The listing builds one solid part. Answer for the finished solid, in the listing's coordinates (mm). A direction names the side the tool comes from. Coordinates: 2 decimals unless noted, no trailing zeros. Write each loop counter-clockwise with the first axis right and the second up, starting at its lowest first coordinate (ties: lowest second). Pieces come first, ordered by that corner, then holes.
from build123d import *

# Parameters (mm, degrees)
BOSS_EXTRUDE1_DEPTH        = 58
SKETCH3_OUTSIDE_W          = 147.986
SKETCH3_OUTSIDE_H          = 126.948
TAB_AND_SLOT_CONTOUR_DEPTH = 3
MOUNTING_TAB_SLOTS_REACH   = 197.382
SKETCH4_W                  = 10.2
SKETCH4_H                  = 4.48444402


with BuildPart() as part:
    # Sketch1 → Boss-Extrude1 (new, symmetric)
    with BuildSketch(Plane.XY):
        Polygon((-63.840100917, 220.738237129), (-95.659428373, 133.315353441), (-98.478506236, 134.341413871), (-66.659178779, 221.764297559), align=None)
    extrude(amount=BOSS_EXTRUDE1_DEPTH, both=True)

    # Sketch3 outside → tab and slot contour (cut)
    with BuildSketch(Plane(origin=(-130.135207504, 47.365341962, 0), x_dir=(0, 0, 1), z_dir=(-0.9396926207859098, 0.3420201433256651, 0))):
        with Locations((0, 139.075)):
            Rectangle(SKETCH3_OUTSIDE_W, SKETCH3_OUTSIDE_H)
        with BuildLine():
            Line((-44.02892944, 185.59149209), (44.02892944, 185.59149209))
            ThreePointArc((44.02892944, 185.59149209), (47.369183029, 184.312070804), (49, 181.128574477))
            Line((49, 181.128574477), (57.97107056, 98.09508485))
            ThreePointArc((57.97107056, 98.09508485), (56.720578714, 94.217748875), (53, 92.558002463))
            Line((53, 92.558002463), (-53, 92.558002463))
            ThreePointArc((-53, 92.558002463), (-56.720578714, 94.217748875), (-57.97107056, 98.09508485))
            Line((-57.97107056, 98.09508485), (-49, 181.128574477))
            ThreePointArc((-49, 181.128574477), (-47.369183029, 184.312070804), (-44.02892944, 185.59149209))
        make_face(mode=Mode.SUBTRACT)
    extrude(amount=-TAB_AND_SLOT_CONTOUR_DEPTH, mode=Mode.SUBTRACT)

    # Sketch4 → mounting tab slots (cut, up to next)
    with BuildSketch(Plane(origin=(-130.135207504, 47.365341962, 0), x_dir=(0, 0, 1), z_dir=(-0.9396926207859099, 0.3420201433256647, 0)), mode=Mode.PRIVATE) as mounting_tab_slots_sk1:
        with Locations((-25, 173.44927008)):
            Rectangle(SKETCH4_W, SKETCH4_H)
    mounting_tab_slots_tool1 = extrude(mounting_tab_slots_sk1.sketch, amount=-MOUNTING_TAB_SLOTS_REACH, mode=Mode.PRIVATE) & part.part
    # Sketch4 → mounting tab slots (cut, up to next)
    with BuildSketch(Plane(origin=(-130.135207504, 47.365341962, 0), x_dir=(0, 0, 1), z_dir=(-0.9396926207859099, 0.3420201433256647, 0)), mode=Mode.PRIVATE) as mounting_tab_slots_sk2:
        with Locations((-25, 103.608313771)):
            Rectangle(SKETCH4_W, SKETCH4_H)
    mounting_tab_slots_tool2 = extrude(mounting_tab_slots_sk2.sketch, amount=-MOUNTING_TAB_SLOTS_REACH, mode=Mode.PRIVATE) & part.part
    # Sketch4 → mounting tab slots (cut, up to next)
    with BuildSketch(Plane(origin=(-130.135207504, 47.365341962, 0), x_dir=(0, 0, 1), z_dir=(-0.9396926207859099, 0.3420201433256647, 0)), mode=Mode.PRIVATE) as mounting_tab_slots_sk3:
        with Locations((25, 173.44927008)):
            Rectangle(SKETCH4_W, SKETCH4_H)
    mounting_tab_slots_tool3 = extrude(mounting_tab_slots_sk3.sketch, amount=-MOUNTING_TAB_SLOTS_REACH, mode=Mode.PRIVATE) & part.part
    # Sketch4 → mounting tab slots (cut, up to next)
    with BuildSketch(Plane(origin=(-130.135207504, 47.365341962, 0), x_dir=(0, 0, 1), z_dir=(-0.9396926207859099, 0.3420201433256647, 0)), mode=Mode.PRIVATE) as mounting_tab_slots_sk4:
        with Locations((25, 103.608313771)):
            Rectangle(SKETCH4_W, SKETCH4_H)
    mounting_tab_slots_tool4 = extrude(mounting_tab_slots_sk4.sketch, amount=-MOUNTING_TAB_SLOTS_REACH, mode=Mode.PRIVATE) & part.part
    add(mounting_tab_slots_tool1.solids().sort_by_distance((-70.812063, 210.354341, -25))[0], mode=Mode.SUBTRACT)
    add(mounting_tab_slots_tool2.solids().sort_by_distance((-94.699077, 144.72531, -25))[0], mode=Mode.SUBTRACT)
    add(mounting_tab_slots_tool3.solids().sort_by_distance((-70.812063, 210.354341, 25))[0], mode=Mode.SUBTRACT)
    add(mounting_tab_slots_tool4.solids().sort_by_distance((-94.699077, 144.72531, 25))[0], mode=Mode.SUBTRACT)


solid = part.part
Q1. The part is cut by section C-C, the plane x = -83. Write down the section's boundary in (y, z).
Answers below:
outline: (168.1, -54.57) - (176.87, -53.68) - (176.87, 53.68) - (168.1, 54.57) - close
Q2. Given pin 1 (5 mm diameter, centred on x = -94, y = 144.5, fed in from -Z); pin 2 (2 mm diameter, centred on x = -94, y = 144.5, fed in from +Z); pin 3 (5 mm diameter, centred on y = 207, z = -44.5, fed in from -X), each flat-ended and moving along its own axis, determine where each tip first touches the part or whether it passes through.
Answers below:
pin 1: stops at z = -57.64
pin 2: stops at z = 57.48
pin 3: stops at x = -72.94
Q3. Find the intervals of material crossed by probe 1 along Z at (x, y) = (-93, 142); probe 2 along X at (y, z) = (192, 44); probe 3 along X at (y, z) = (144, -32.5), in increasing order.
Answers below:
probe 1: z = -57.59 to -30.1, -19.9 to 19.9, 30.1 to 57.59
probe 2: x = -77.49 to -74.3
probe 3: x = -94.96 to -91.77
Q4. Which of the six approach directions +Z, -Z, +X, -X, +Y, -Y give full straight-line access (tool end or side, diameter ignored) to faces 1 (the face through (-80.797, 178.598, 53.423)), 2 (the face through (-81.194, 177.506, -53.548)), 3 (the face through (-68.655, 211.955, 24.929)), 4 (the face through (-94.076, 142.112, 24.929)), 5 (the face through (-93, 144, -30.1))?
Answers below:
face 1: +Z, +X, +Y
face 2: -Z, +X, +Y
face 3: -X
face 4: +X
face 5: none
Q5. The part is cut by section D-D, the plane z = -6.5. Write down the section's boundary in (x, y), then the cut area to 3 significant figures.
Answers below:
outline: (-98.48, 134.34) - (-95.66, 133.32) - (-63.84, 220.74) - (-66.66, 221.76) - close
area: 279 mm2
Q6. The part is cut by section B-B, the plane y = 210. Write down the section's boundary in (x, z).
Answers below:
outline: (-70.94, -49.87) - (-67.75, -49.75) - (-67.75, -30.1) - (-70.94, -30.1) - close; (-70.94, -19.9) - (-67.75, -19.9) - (-67.75, 19.9) - (-70.94, 19.9) - close; (-70.94, 30.1) - (-67.75, 30.1) - (-67.75, 49.75) - (-70.94, 49.87) - close
Q7. Determine the mould class of faces 6 (the face through (-92.542, 146.326, -25.071)), 7 (the face through (-97.089, 133.836, 0.742)), 8 (the face through (-82.79, 177.44, 0.81)) for opening direction Y: released by +Y, released by -Y, zero draft, split by the parting line, or undercut.
Answers below:
face 6: undercut
face 7: released by -Y
face 8: released by +Y
Q8. The part is cut by section A-A, the plane z = 22.5. Write down the section's boundary in (x, y).
Answers below:
outline: (-98.48, 134.34) - (-95.66, 133.32) - (-92.65, 141.59) - (-95.47, 142.62) - close; (-93.93, 146.83) - (-91.11, 145.81) - (-68.76, 207.22) - (-71.58, 208.25) - close; (-70.05, 212.46) - (-67.23, 211.44) - (-63.84, 220.74) - (-66.66, 221.76) - close
